from build123d import *

# Parameters (mm, degrees)
F0_R     = 7.5
F0_R_2   = 37.5
F1_DEPTH = 5
F0_R_3   = 35
F2_DEPTH = 70


with BuildPart() as f1:
    # F0 (on Front) → F1 (new body, symmetric)
    with BuildSketch(Plane.XZ):
        with BuildLine():
            ThreePointArc((150, 55), (144.1421356237, 69.1421356237), (130, 75))
            Line((130, 75), (-130, 75))
            ThreePointArc((-130, 75), (-144.1421356237, 69.1421356237), (-150, 55))
            Line((-150, 55), (-150, -55))
            ThreePointArc((-150, -55), (-144.1421356237, -69.1421356237), (-130, -75))
            Line((-130, -75), (130, -75))
            ThreePointArc((130, -75), (144.1421356237, -69.1421356237), (150, -55))
            Line((150, -55), (150, 55))
        make_face()
        with Locations((-130, -55)):
            Circle(F0_R, mode=Mode.SUBTRACT)
        with Locations((130, -55)):
            Circle(F0_R, mode=Mode.SUBTRACT)
        with Locations((-130, 55)):
            Circle(F0_R, mode=Mode.SUBTRACT)
        Circle(F0_R_2, mode=Mode.SUBTRACT)
        with Locations((130, 55)):
            Circle(F0_R, mode=Mode.SUBTRACT)
    extrude(amount=F1_DEPTH, both=True)

    # F0 (on Front) → F2 (join)
    with BuildSketch(Plane.XZ):
        Circle(F0_R_2)
        Circle(F0_R_3, mode=Mode.SUBTRACT)
    extrude(amount=F2_DEPTH)


solid = f1.part
Work out the finished part from the listing and answer in its coordinate system (mm). A direction names the side the tool comes from. Give positions to 0.01 mm unless a question says otherwise; leave off trailing zeros. Loops run counter-clockwise (first coordinate to the right, second up) from the corner with the lowest first, then second, coordinate; pieces in that order, holes last. Notation, with made-up numbers: (3, 49.5) - (30, 49.5) arc R12 cw to (30, 68.5) - close; hole circle Ø2 at (25.25, -31.75). An arc over 180 degrees is marked (long way). Answer in a Markdown table with one row per item. Add a question column.
Q1. The part is cut by section A-A (z = 0). Determine the outline of the cut face in (x, y).
Q2. The part is cut by section C-C (z = 50.5). Determine the outline of the cut face in (x, y).
Q3. The part is cut by section D-D (y = -9.5). Determine the outline of the cut face in (x, z).
Q4. Each of these flat-tipped pins is pushed along its axis until it touches: P1, Ø3, axis at x = 30.5, y = -57.5, coming from the +Z side (3 decimals); P2, Ø1, axis at x = 48.5, z = 54, coming from the -Y side; P3, Ø5, axis at y = -54.5, z = 12.5, coming from the -X side. Where does it stop, or does it pass through?
Q5. The part is cut by section B-B (x = 0). Determine the outline of the cut face in (y, z), and give its area (3 significant figures).
Q6. Consider line 1 along Z through (x, y) = (-130, 3.25); line 2 along Z through (x, y) = (0, -52.5); line 3 along X through (y, z) = (0, -57). Determine where each line is inside the solid, lowest interval first.
Q7. A tool of negligible diameter and unlimited length cuts with its end or side. For faces 1 (the cylindrical face through (-4.88, 2.54, 37.18)), 2 (the flat face through (-35, -5, -16)), 3 (the flat face through (-2, 0, -75)), from which of +Z, -Z, +X, -X, +Y, -Y can it reach the whole face along a straight path? Write none if from no direction.
Q8. Determine the mould class of faces 4 (the cylindrical face through (136.93, 0.07, -57.87)), 5 (the cylindrical face through (-4.88, -37.04, 37.18)), 6 (the flat face through (150, 0, -1)) for opening direction X: released by +X, released by -X, zero draft, split by the parting line, or undercut.
Solution:
| question | item | result |
|---|---|---|
| 1 | outline | (-150, -5) - (-37.5, -5) - (-37.5, -70) - (-35, -70) - (-35, 0) - (-37.5, 0) - (-37.5, 5) - (-150, 5) - close; (35, -70) - (37.5, -70) - (37.5, -5) - (150, -5) - (150, 5) - (37.5, 5) - (37.5, 0) - (35, 0) - close |
| 2 | outline | (-150, -5) - (-136, -5) - (-136, 5) - (-150, 5) - close; (-124, -5) - (124, -5) - (124, 5) - (-124, 5) - close; (136, -5) - (150, -5) - (150, 5) - (136, 5) - close |
| 3 | outline | circle Ø75 at (0, 0); hole circle Ø70 at (0, 0) |
| 4 | P1 | stops at z = 23.775 |
| 4 | P2 | stops at y = -5 |
| 4 | P3 | stops at x = -36.14 |
| 5 | outline | (-70, -37.5) - (-5, -37.5) - (-5, -75) - (5, -75) - (5, -37.5) - (0, -37.5) - (0, -35) - (-70, -35) - close; (-70, 35) - (0, 35) - (0, 37.5) - (5, 37.5) - (5, 75) - (-5, 75) - (-5, 37.5) - (-70, 37.5) - close |
| 5 | area | 1,100 mm² |
| 6 | line 1 | z = -75 to -62.5, -47.5 to 47.5, 62.5 to 75 |
| 6 | line 2 | z = -37.5 to -35, 35 to 37.5 |
| 6 | line 3 | x = -149.9 to -137.23, -122.77 to 122.77, 137.23 to 149.9 |
| 7 | face 1 | +Y |
| 7 | face 2 | -Y |
| 7 | face 3 | -Z, +X, -X, +Y, -Y |
| 8 | face 4 | undercut |
| 8 | face 5 | split by the parting line |
| 8 | face 6 | released by +X |
